from build123d import *

# Parameters (mm, degrees)
F1_DEPTH = 191.008
F2_R     = 1.27


with BuildPart() as f1:
    # F0 (on Right) → F1 (new body)
    with BuildSketch(Plane.YZ):
        Polygon((0, 44.9834), (0, 0), (42.672, 0), (42.672, 44.9834), (45.3136, 44.9834), (39.497, 50.8), (39.497, 3.175), (3.175, 3.175), (3.175, 50.8), (-2.6416, 44.9834), align=None)
    extrude(amount=F1_DEPTH)

    # F2
    f2_edges = [f1.edges().sort_by_distance(p)[0] for p in [
        (95.504, 3.175, 50.8),
        (95.504, 39.497, 50.8),
    ]]
    fillet(f2_edges, radius=F2_R)


solid = f1.part
Read the model definition and answer for the solid it produces. Units are mm, in the model's axes. A direction names the side the tool comes from. Round coordinates to 2 decimals unless told otherwise and drop trailing zeros. Order: outer loops, then holes, each group sorted by start corner. A loop starts at its lowest first (then second) coordinate and runs counter-clockwise, first axis right, second up. Notation, with made-up numbers: (11, 58) - (38, 58) arc R27 cw to (38, 80) - close; hole circle Ø3 at (-18, 58.25). An arc over 180 degrees is marked (long way). Use one line per item in the form item = value. Start each with the question number.
(1) Flat-ended cylindrical pins translate along their axes: pin 1 Ø6 at (x, y) = (63, 10) entering from +Z (3 decimals); pin 2 Ø13.5 at (x, z) = (65.5, 28) entering from -Y; pin 3 Ø6 at (x, z) = (74.5, 30.5) entering from +Y. Find the tip coordinate at first contact, or state that the pin passes through.
(2) The part is cut by section B-B (z = 5.5). Give the vertices of the cut face in (x, y) (3 decimals).
(3) Determine the mould class of faces 4 (the face through (94, 42.672, 22)), 5 (the face through (94, 21, 0)), 6 (the face through (94, 22, 3.175)) for opening direction Y: +Y half, -Y half, draft (parallel to the pull), parting line (faces both ways), or undercut.
(4) The part is cut by section A-A (x = 98). Give the vertices of the cut face in (y, z) (3 decimals), then the cut area to 3 significant figures.
(5) The part is cut by section C-C (y = 16.5). Give the vertices of the cut face in (x, z) (3 decimals), then the cut area to 3 significant figures.
(6) Find the intervals of material crossed by line 1 along Y through (x, z) = (51, 16) (3 decimals); line 2 along Z through (x, y) = (95.5, 29.5) (3 decimals); line 3 along Z through (x, y) = (47.5, 3), in increasing order. Write a range as from..to.
(7) For faces 1 (the face through (0, 25, 3)), 2 (the face through (94, 0, 23)), 3 (the face through (94, 3.175, 25)), determine the directions among +Z, -Z, +X, -X, +Y, -Y from which every point of the face is accessible in a straight line to the end or side of a thin tool.
Checked values:
q1.pin_1 = 3.175
q1.pin_2 = 0
q1.pin_3 = 42.67
q2.outline = (0, 0) - (191.008, 0) - (191.008, 3.175) - (0, 3.175) - close; (0, 39.497) - (191.008, 39.497) - (191.008, 42.672) - (0, 42.672) - close
q3.face_4 = +Y half
q3.face_5 = draft
q3.face_6 = undercut
q4.outline = (-2.642, 44.983) - (0, 44.983) - (0, 0) - (42.672, 0) - (42.672, 44.983) - (45.314, 44.983) - (41.665, 48.632) arc R1.27 ccw to (39.497, 47.734) - (39.497, 3.175) - (3.175, 3.175) - (3.175, 47.734) arc R1.27 ccw to (1.007, 48.632) - close
q4.area = 431 mm^2
q5.outline = (0, 0) - (191.008, 0) - (191.008, 3.175) - (0, 3.175) - close
q5.area = 606 mm^2
q6.line_1 = 0..3.175, 39.497..42.672
q6.line_2 = 0..3.175
q6.line_3 = 0..48.38
q7.face_1 = +Z, -Z, -X, +Y, -Y
q7.face_2 = -Z, +X, -X, -Y
q7.face_3 = +Z, +X, -X
